Here's how the part is built. I have some questions about the finished solid (model axes, mm). Face numbers are marked on the shaded views. A direction names the side the tool comes from. Round coordinates to 2 decimals unless told otherwise and drop trailing zeros. Write each loop counter-clockwise with the first axis right and the second up, starting at its lowest first coordinate (ties: lowest second). Pieces come first, ordered by that corner, then holes. Notation, with made-up numbers: (51.25, 9.25) - (74.25, 9.25) arc R23 ccw to (74.25, 26.25) - close; hole circle Ø6 at (58, 15). An arc over 180 degrees is marked (long way). Write item = value, one per line. Start each with the question number.
Item 1: If we section it at D-D (z = 14.5): Please give me the cut outline in (x, y), and give its area (3 significant figures).
Item 2: If I drill on line 1 along Z through (x, y) = (-6, 1.8); line 2 along Y through (x, z) = (-7, 14.5); line 3 along Z through (x, y) = (-1.5, 2.5), over which ranges is the centre line in solid material (lowest first)? Write a range as [from, to].
Item 3: If we section it at B-B (z = 18.25): Please give me the cut outline in (x, y).
Item 4: For P1, Ø6, axis at x = 6, z = 9, coming from the +Y side; P2, Ø5, axis at x = 26.5, z = 11.5, coming from the +Y side; P3, Ø7, axis at x = -6, z = 10, coming from the +Y side, each with a flat end and sliding along its axis, tell me the tip position at first contact or that it passes through.
Item 5: Which directions (+Z, -Z, +X, -X, +Y, -Y) give clear straight access to the entire face, cutting with the end or side of a thin tool? Please do the marked faces 1, 2 and 3.
Item 6: Thinking about a two-plate mould opening in X: for the marked faces 4, 5, 6 and 7, which applies, pulls with the +X half, pulls with the -X half, needs draft (parallel to the pull), parting line crosses it, or undercut?
Item 7: If we section it at C-C (x = 26): Please give me the cut outline in (y, z).
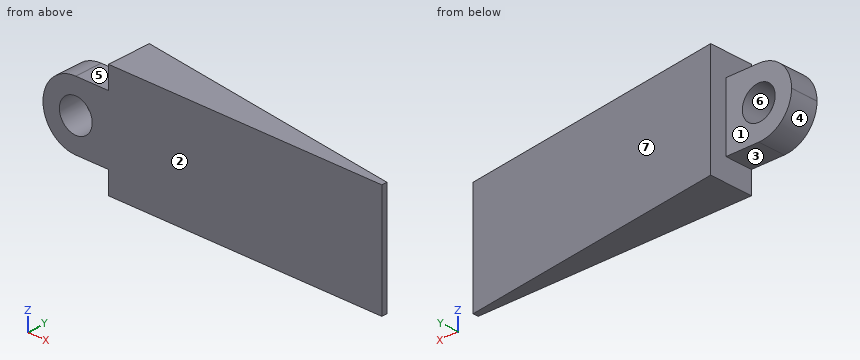
```python
from build123d import *

# Parameters (mm, degrees)
PAD_DEPTH    = 20
SKETCH001_W  = 5
SKETCH001_H  = 12
PAD001_DEPTH = 12
FILLET_R     = 5.99
SKETCH002_R  = 3
POCKET_DEPTH = 5


with BuildPart() as part:
    # Sketch → Pad (new body)
    with BuildSketch(Plane.XY):
        Polygon((0, 0), (50, 0), (50, 1), (0, 8), align=None)
    extrude(amount=PAD_DEPTH)

    # Sketch001 → Pad001 (new body)
    with BuildSketch(Plane(origin=(0, 0, 0), x_dir=(0, -1, 0), z_dir=(-1, 0, 0))):
        with Locations((-2.5, 10)):
            Rectangle(SKETCH001_W, SKETCH001_H)
    extrude(amount=PAD001_DEPTH)

    # Fillet
    fillet_edges = [part.edges().sort_by_distance(p)[0] for p in [
        (-12, 2.5, 16),
        (-12, 2.5, 4),
    ]]
    fillet(fillet_edges, radius=FILLET_R)

    # Sketch002 → Pocket (cut)
    with BuildSketch(Plane(origin=(0, 5, 0), x_dir=(-1, 0, 0), z_dir=(0, 1, 0))):
        with Locations((6, 10)):
            Circle(SKETCH002_R)
    extrude(amount=-POCKET_DEPTH, mode=Mode.SUBTRACT)


solid = part.part
```
Reply:
q1.outline = (-9.97, 0) - (50, 0) - (50, 1) - (0, 8) - (0, 5) - (-9.97, 5) - close
q1.area = 275 mm2
q2.line_1 = [4, 7], [13, 16]
q2.line_2 = [0, 5]
q2.line_3 = [4, 16]
q3.outline = (0, 0) - (50, 0) - (50, 1) - (0, 8) - close
q4.P1 = 7.58
q4.P2 = 4.64
q4.P3 = 5
q5.face_1 = +Z, -Z, -X, +Y
q5.face_2 = +Z, -Z, +X, -X, -Y
q5.face_3 = -Z, -X, +Y, -Y
q6.face_4 = pulls with the -X half
q6.face_5 = needs draft
q6.face_6 = undercut
q6.face_7 = pulls with the +X half
q7.outline = (0, 0) - (4.36, 0) - (4.36, 20) - (0, 20) - close
